Read the model definition and answer for the solid it produces. Units are mm, in the model's axes. A direction names the side the tool comes from. Round coordinates to 2 decimals unless told otherwise and drop trailing zeros. Order: outer loops, then holes, each group sorted by start corner. A loop starts at its lowest first (then second) coordinate and runs counter-clockwise, first axis right, second up. Notation, with made-up numbers: M 39.5,28 L 56.5,28 A15 cw 56.5,45 Z; hole C -9,35.25 d3. An arc over 180 degrees is marked long. Answer as CSV lines item,"result".
```python
from build123d import *

# Parameters (mm, degrees)
F0_W        = 44
F0_H        = 61
F1_DEPTH    = 2
F3_DEPTH    = 7
F4_R        = 3
F4_R_2      = 1.5
F5_DEPTH    = 5
F6_T4_DEPTH = 44
F7_W        = 44
F7_H        = 4.4
F8_DEPTH    = 7
F9_R        = 1.5
F10_DEPTH   = 7
F12_DEPTH   = 2.001


# Not quite as in the source:
# - a fillet or chamfer that OpenCascade refuses, or shapes differently, is made with other operations: its cross-section is extruded or revolved along the edge and cut away or added


with BuildPart() as f1:
    # F0 (on Top) → F1 (new body)
    with BuildSketch(Plane.XY):
        Rectangle(F0_W, F0_H)
    extrude(amount=F1_DEPTH)

    # F2 (on face) → F3 (join)
    with BuildSketch(Plane(origin=(0, 0, 0), x_dir=(1, 0, 0), z_dir=(0, 0, -1))):
        with BuildLine():
            Line((-13.0117940697, 45.5), (-22, 30.5))
            Line((-22, 30.5), (22, 30.5))
            Line((22, 30.5), (13.0117940697, 45.5))
            Line((13.0117940697, 45.5), (4.5, 45.5))
            ThreePointArc((4.5, 45.5), (0, 38.660928057), (-4.5, 45.5))
            Line((-4.5, 45.5), (-13.0117940697, 45.5))
        make_face()
    extrude(amount=-F3_DEPTH)

    # F4 (on face) → F5 (join)
    with BuildSketch(Plane.XY.offset(2)):
        with Locations((-16.9, 22.9)):
            Circle(F4_R)
        with Locations((-16.9, 22.9)):
            Circle(F4_R_2, mode=Mode.SUBTRACT)
        with Locations((16.9, 22.9)):
            Circle(F4_R)
        with Locations((16.9, 22.9)):
            Circle(F4_R_2, mode=Mode.SUBTRACT)
        with Locations((16.9, -22.9)):
            Circle(F4_R)
        with Locations((16.9, -22.9)):
            Circle(F4_R_2, mode=Mode.SUBTRACT)
        with Locations((-16.9, -22.9)):
            Circle(F4_R)
        with Locations((-16.9, -22.9)):
            Circle(F4_R_2, mode=Mode.SUBTRACT)
    extrude(amount=F5_DEPTH)

    # F6: chamfer of 5 on 1 edges, made by hand


with BuildPart() as f6_tool2:
    # F6_s3 → F6_t4 (new body)
    with BuildSketch(Plane.YZ.offset(-22)):
        Polygon((-25.5, 2), (-30.5, 7), (-30.5, 2), align=None)
    extrude(amount=F6_T4_DEPTH)

    split(bisect_by=Plane(origin=(29.6352662025, -17.7578583619, 0), x_dir=(0, 0, 1), z_dir=(-0.8577903364, 0.5139997459, 0)), keep=Keep.TOP)

    split(bisect_by=Plane.XY.offset(7), keep=Keep.BOTTOM)

    split(bisect_by=Plane(origin=(-29.6352662025, -17.7578583619, 0), x_dir=(0, 0, 1), z_dir=(0.8577903364, 0.5139997459, 0)), keep=Keep.TOP)


with BuildPart() as f1_1:
    add(f1.part)

    # F6_t1: union F6_tool2
    add(f6_tool2.part)

    # F7 (on face) → F8 (join)
    with BuildSketch(Plane.XY.offset(2)):
        with Locations((0, 28.3)):
            Rectangle(F7_W, F7_H)
    extrude(amount=F8_DEPTH)

    # F9 (on face) → F10 (cut)
    with BuildSketch(Plane.XY.offset(9)):
        with Locations((-19, 28.3)):
            Circle(F9_R)
        with Locations((19, 28.3)):
            Circle(F9_R)
    extrude(amount=-F10_DEPTH, mode=Mode.SUBTRACT)

    # F11 (on face) → F12 (cut, through all)
    with BuildSketch(Plane.XY.offset(2)):
        with BuildLine():
            Line((16.4316767252, 1.5), (18.9406969249, 1.5))
            ThreePointArc((18.9406969249, 1.5), (13.4350288425, 13.4350288425), (1.5, 18.9406969249))
            Line((1.5, 18.9406969249), (1.5, 16.4316767252))
            ThreePointArc((1.5, 16.4316767252), (11.6672618896, 11.6672618896), (16.4316767252, 1.5))
        make_face()
        with BuildLine():
            ThreePointArc((1.5, -18.9406969249), (13.4350288425, -13.4350288425), (18.9406969249, -1.5))
            Line((18.9406969249, -1.5), (16.4316767252, -1.5))
            ThreePointArc((16.4316767252, -1.5), (11.6672618896, -11.6672618896), (1.5, -16.4316767252))
            Line((1.5, -16.4316767252), (1.5, -18.9406969249))
        make_face()
        with BuildLine():
            Line((-1.5, 16.4316767252), (-1.5, 18.9406969249))
            ThreePointArc((-1.5, 18.9406969249), (-13.4350288425, 13.4350288425), (-18.9406969249, 1.5))
            Line((-18.9406969249, 1.5), (-16.4316767252, 1.5))
            ThreePointArc((-16.4316767252, 1.5), (-11.6672618896, 11.6672618896), (-1.5, 16.4316767252))
        make_face()
        with BuildLine():
            Line((11.401754251, 1.5), (13.9194109071, 1.5))
            ThreePointArc((13.9194109071, 1.5), (9.8994949366, 9.8994949366), (1.5, 13.9194109071))
            Line((1.5, 13.9194109071), (1.5, 11.401754251))
            ThreePointArc((1.5, 11.401754251), (8.1317279836, 8.1317279836), (11.401754251, 1.5))
        make_face()
        with BuildLine():
            ThreePointArc((-18.9406969249, -1.5), (-13.4350288425, -13.4350288425), (-1.5, -18.9406969249))
            Line((-1.5, -18.9406969249), (-1.5, -16.4316767252))
            ThreePointArc((-1.5, -16.4316767252), (-11.6672618896, -11.6672618896), (-16.4316767252, -1.5))
            Line((-16.4316767252, -1.5), (-18.9406969249, -1.5))
        make_face()
        with BuildLine():
            ThreePointArc((1.5, -13.9194109071), (9.8994949366, -9.8994949366), (13.9194109071, -1.5))
            Line((13.9194109071, -1.5), (11.401754251, -1.5))
            ThreePointArc((11.401754251, -1.5), (8.1317279836, -8.1317279836), (1.5, -11.401754251))
            Line((1.5, -11.401754251), (1.5, -13.9194109071))
        make_face()
        with BuildLine():
            Line((-1.5, 11.401754251), (-1.5, 13.9194109071))
            ThreePointArc((-1.5, 13.9194109071), (-9.8994949366, 9.8994949366), (-13.9194109071, 1.5))
            Line((-13.9194109071, 1.5), (-11.401754251, 1.5))
            ThreePointArc((-11.401754251, 1.5), (-8.1317279836, 8.1317279836), (-1.5, 11.401754251))
        make_face()
        with BuildLine():
            Line((6.3245553203, 1.5), (8.8741196746, 1.5))
            ThreePointArc((8.8741196746, 1.5), (6.3639610307, 6.3639610307), (1.5, 8.8741196746))
            Line((1.5, 8.8741196746), (1.5, 6.3245553203))
            ThreePointArc((1.5, 6.3245553203), (4.5961940777, 4.5961940777), (6.3245553203, 1.5))
        make_face()
        with BuildLine():
            ThreePointArc((-13.9194109071, -1.5), (-9.8994949366, -9.8994949366), (-1.5, -13.9194109071))
            Line((-1.5, -13.9194109071), (-1.5, -11.401754251))
            ThreePointArc((-1.5, -11.401754251), (-8.1317279836, -8.1317279836), (-11.401754251, -1.5))
            Line((-11.401754251, -1.5), (-13.9194109071, -1.5))
        make_face()
        with BuildLine():
            ThreePointArc((1.5, -8.8741196746), (6.3639610307, -6.3639610307), (8.8741196746, -1.5))
            Line((8.8741196746, -1.5), (6.3245553203, -1.5))
            ThreePointArc((6.3245553203, -1.5), (4.5961940777, -4.5961940777), (1.5, -6.3245553203))
            Line((1.5, -6.3245553203), (1.5, -8.8741196746))
        make_face()
        with BuildLine():
            Line((-1.5, 6.3245553203), (-1.5, 8.8741196746))
            ThreePointArc((-1.5, 8.8741196746), (-6.3639610307, 6.3639610307), (-8.8741196746, 1.5))
            Line((-8.8741196746, 1.5), (-6.3245553203, 1.5))
            ThreePointArc((-6.3245553203, 1.5), (-4.5961940777, 4.5961940777), (-1.5, 6.3245553203))
        make_face()
        with BuildLine():
            Line((1.5, 1.5), (3.7080992435, 1.5))
            ThreePointArc((3.7080992435, 1.5), (2.8284271247, 2.8284271247), (1.5, 3.7080992435))
            Line((1.5, 3.7080992435), (1.5, 1.5))
        make_face()
        with BuildLine():
            ThreePointArc((-8.8741196746, -1.5), (-6.3639610307, -6.3639610307), (-1.5, -8.8741196746))
            Line((-1.5, -8.8741196746), (-1.5, -6.3245553203))
            ThreePointArc((-1.5, -6.3245553203), (-4.5961940777, -4.5961940777), (-6.3245553203, -1.5))
            Line((-6.3245553203, -1.5), (-8.8741196746, -1.5))
        make_face()
        with BuildLine():
            ThreePointArc((1.5, -3.7080992435), (2.8284271247, -2.8284271247), (3.7080992435, -1.5))
            Line((3.7080992435, -1.5), (1.5, -1.5))
            Line((1.5, -1.5), (1.5, -3.7080992435))
        make_face()
        with BuildLine():
            Line((-1.5, 1.5), (-1.5, 3.7080992435))
            ThreePointArc((-1.5, 3.7080992435), (-2.8284271247, 2.8284271247), (-3.7080992435, 1.5))
            Line((-3.7080992435, 1.5), (-1.5, 1.5))
        make_face()
        with BuildLine():
            ThreePointArc((-1.03e-08, -1.5), (1.0606601681, -1.0606601754), (1.5, 0))
            ThreePointArc((1.5, 0), (1.0606601718, 1.0606601718), (0, 1.5))
            ThreePointArc((0, 1.5), (-1.0606601711, 1.0606601725), (-1.5, 2e-09))
            ThreePointArc((-1.5, 2e-09), (-1.0606601761, -1.0606601674), (-1.03e-08, -1.5))
        make_face()
        with BuildLine():
            ThreePointArc((-3.7080992435, -1.5), (-2.8284271247, -2.8284271247), (-1.5, -3.7080992435))
            Line((-1.5, -3.7080992435), (-1.5, -1.5))
            Line((-1.5, -1.5), (-3.7080992435, -1.5))
        make_face()
    extrude(amount=-F12_DEPTH, mode=Mode.SUBTRACT)


solid = f1_1.part
```
Item 1: A cutting plane is placed at B-B, the plane y = 22.9. Determine the outline of the cut face in (x, z), and give its area (3 significant figures).
Ans:
outline,"M -22,0 L 22,0 L 22,2 L 19.9,2 L 19.9,7 L 18.4,7 L 18.4,2 L 15.4,2 L 15.4,7 L 13.9,7 L 13.9,2 L -13.9,2 L -13.9,7 L -15.4,7 L -15.4,2 L -18.4,2 L -18.4,7 L -19.9,7 L -19.9,2 L -22,2 Z"
area,"118 mm2"
Item 2: A tool of negligible diameter and unlimited length cuts with its end or side. For faces 1 (the face through (0, 26.1, 5)), 2 (the face through (-5, 1, 2)), 3 (the face through (0, 30.5, 4)), 4 (the face through (13, 1.5, 1)), from which of +Z, -Z, +X, -X, +Y, -Y can it reach the whole face along a straight path? Write none if from no direction.
Ans:
face 1,"+Z, +X, -X"
face 2,"+Z"
face 3,"+Z, -Z, +X, -X, +Y"
face 4,"+Z, -Z"
Item 3: Determine the mould class of faces 5 (the face through (-0.3, -28, 4.5)), 6 (the face through (9, -45.5, 3)), 7 (the face through (-22, 2.1, 1.8)) for opening direction Y: +Y half, -Y half, draft (parallel to the pull), parting line (faces both ways), or undercut.
Ans:
face 5,"undercut"
face 6,"-Y half"
face 7,"draft"
Item 4: A cutting plane is placed at A-A, the plane z = 6.25. Give the number of separate pieces and of enclosed holes in the cut face, and give its area (3 significant figures).
Ans:
separate pieces,"6"
enclosed holes,"6"
area,"766 mm2"
Item 5: A cutting plane is placed at D-D, the plane y = -32.5. Determine the outline of the cut face in (x, z).
Ans:
outline,"M -20.8,0 L 20.8,0 L 20.8,7 L -20.8,7 Z"
Item 6: Flat-ended cylindrical pins translate along their axes: pin 1 (1.5 mm diameter, centred on x = 16.5, y = -22.5, fed in from +Z); pin 2 (10 mm diameter, centred on x = 1.5, y = -25, fed in from -Z); pin 3 (3 mm diameter, centred on y = -34.5, z = 4, fed in from +X); pin 4 (0.6 mm diameter, centred on x = 3, z = 1, fed in from -Y). Find the tip coordinate at first contact, or state that the pin passes through.
Ans:
pin 1,"z = 2"
pin 2,"z = 0"
pin 3,"x = 20.5"
pin 4,"y = -39.94"
Item 7: Find the intervals of material crossed by probe 1 along Y at (x, z) = (14.5, 1.75); probe 2 along Y at (x, z) = (-19, 5.5); probe 3 along X at (y, z) = (-22.5, 4.75), in increasing order. Write a range as [from, to].
Ans:
probe 1,"[-43.02, -12.28], [-7.87, 7.87], [12.28, 30.5]"
probe 2,"[-35.51, -29], [-25.04, -20.76], [20.76, 25.04], [26.1, 26.8], [29.8, 30.5]"
probe 3,"[-19.87, -18.35], [-15.45, -13.93], [13.93, 15.45], [18.35, 19.87]"
